Can you work these out from the model? Positions are in its coordinate system, mm. A direction names the side the tool comes from. Give positions to 0.01 mm unless a question says otherwise; leave off trailing zeros. Order: outer loops, then holes, each group sorted by start corner. A loop starts at its lowest first (then second) coordinate and runs counter-clockwise, first axis right, second up. Notation, with made-up numbers: (-16.75, 85) -> (32.25, 85) arc R7 cw to (32.25, 97) -> close; hole circle Ø9 at (-38, 74.25). An arc over 180 degrees is marked (long way). Answer as a JSON object with one key per item and string values.
```python
from build123d import *

# Parameters (mm, degrees)
SKETCH1_W           = 162.5727
SKETCH1_H           = 69.9897
BOSS_EXTRUDE1_DEPTH = 101.6635
SKETCH2_R           = 9.525
BOSS_EXTRUDE2_DEPTH = 69.9897
SKETCH3_W           = 34.9885
SKETCH3_H           = 22.29485
CUT_EXTRUDE1_DEPTH  = 1275.884686052
CUT_EXTRUDE2_DEPTH  = 27.432
CUT_EXTRUDE3_REACH  = 1269.087
CUT_EXTRUDE5_REACH  = 1269.087


with BuildPart() as part:
    # Sketch1 → Boss-Extrude1 (new body)
    with BuildSketch(Plane.XY):
        with Locations((634.389537826, 1225.388271401)):
            Rectangle(SKETCH1_W, SKETCH1_H)
    extrude(amount=BOSS_EXTRUDE1_DEPTH)

    # Sketch2 → Boss-Extrude2 (add, through all)
    with BuildSketch(Plane(origin=(0, 1260.383121401, 0), x_dir=(1, 0, 0), z_dir=(0, 1, 0))):
        Polygon((582.567187826, 0), (625.213787826, 34.9885), (643.565287826, 34.9885), (686.211887826, 0), align=None)
        with Locations(Location((634.389537826, 15.3035, 0), (0, 0, 270))):
            Circle(SKETCH2_R, mode=Mode.SUBTRACT)
    extrude(amount=-BOSS_EXTRUDE2_DEPTH)

    # Sketch3 → Cut-Extrude1 (cut, through all)
    with BuildSketch(Plane.ZY.offset(-553.103187826)):
        with Locations((-17.49425, 1201.540846401)):
            Rectangle(SKETCH3_W, SKETCH3_H)
        with Locations((-17.49425, 1249.235696401)):
            Rectangle(SKETCH3_W, SKETCH3_H)
    extrude(amount=-CUT_EXTRUDE1_DEPTH, mode=Mode.SUBTRACT)

    # Sketch5 → Cut-Extrude2 (cut, symmetric)
    with BuildSketch(Plane(origin=(0, 1225.388271401, 0), x_dir=(1, 0, 0), z_dir=(0, 1, 0))):
        Polygon((558.183187826, -101.6635), (561.485187826, -91.5035), (707.293887826, -91.5035), (710.595887826, -101.6635), align=None)
    extrude(amount=CUT_EXTRUDE2_DEPTH, both=True, mode=Mode.SUBTRACT)

    # Cut-Extrude3: up to this plane
    cut_extrude3_end = Plane(origin=(707.293887826, 1197.956271401, 91.5035), z_dir=(0.9510340687309474, 0, -0.3090860723375604))
    # Sketch6 → Cut-Extrude3 (cut, up to the surface)
    with BuildSketch(Plane.ZY.offset(-634.389537826), mode=Mode.PRIVATE) as cut_extrude3_sk1:
        Polygon((101.6635, 1255.303121401), (91.5035, 1252.820271401), (101.6635, 1252.820271401), align=None)
    cut_extrude3_tool1 = split(extrude(cut_extrude3_sk1.sketch, amount=-CUT_EXTRUDE3_REACH, mode=Mode.PRIVATE), bisect_by=cut_extrude3_end, keep=Keep.BOTH, mode=Mode.PRIVATE)
    add(cut_extrude3_tool1.solids().sort_by_distance((634.389538, 1253.647888, 98.276833))[0], mode=Mode.SUBTRACT)
    # Sketch6 → Cut-Extrude3 (cut, up to the surface)
    with BuildSketch(Plane.ZY.offset(-634.389537826), mode=Mode.PRIVATE) as cut_extrude3_sk2:
        Polygon((91.5035, 1197.956271401), (101.6635, 1195.473421401), (101.6635, 1197.956271401), align=None)
    cut_extrude3_tool2 = split(extrude(cut_extrude3_sk2.sketch, amount=-CUT_EXTRUDE3_REACH, mode=Mode.PRIVATE), bisect_by=cut_extrude3_end, keep=Keep.BOTH, mode=Mode.PRIVATE)
    add(cut_extrude3_tool2.solids().sort_by_distance((634.389538, 1197.128655, 98.276833))[0], mode=Mode.SUBTRACT)

    # Cut-Extrude5: up to this face of the body (flat: up to its plane)
    cut_extrude5_end = Plane(part.part.faces().sort_by_distance((559.834187826, 1225.388271401, 96.5835))[0])
    # Sketch8 → Cut-Extrude5 (cut, up to the picked face)
    with BuildSketch(Plane(origin=(634.389537826, 0, 0), x_dir=(0, 0, -1), z_dir=(1, 0, 0)), mode=Mode.PRIVATE) as cut_extrude5_sk1:
        Polygon((-101.6635, 1255.303121401), (-91.5035, 1252.820271401), (-91.5035, 1197.956271401), (-101.6635, 1195.473421401), align=None)
    cut_extrude5_tool1 = split(extrude(cut_extrude5_sk1.sketch, amount=-CUT_EXTRUDE5_REACH, mode=Mode.PRIVATE), bisect_by=cut_extrude5_end, keep=Keep.BOTH, mode=Mode.PRIVATE)
    add(cut_extrude5_tool1.solids().sort_by(Axis((634.389538, 1225.388271, 96.656813), (-1, 0, 0)))[0], mode=Mode.SUBTRACT)


solid = part.part
```
1. For faces 1 (the face through (645, 1212.688, -14)), 2 (the face through (645, 1238.088, -14)), 3 (the face through (640.83, 1225.57, -22.32)), 4 (the face through (708.92, 1224.97, 96.51)), which set-ups out of +Z, -Z, +X, -X, +Y, -Y let a thin tool reach every point of the face, with its end or its side?
Worked answers:
{"face 1": "-Z, +X, -X, -Y", "face 2": "-Z, +X, -X, +Y", "face 3": "+Y, -Y", "face 4": "+Z"}
2. If we mould it in two halves opening along Y, with no side actions, what happens to faces 5 (the face through (553.103, 1225, 50)), 6 (the face through (635.456, 1196.732, 96.512)), 7 (the face through (633, 1190.393, 50))? For each: +Y half, -Y half, draft (parallel to the pull), parting line (faces both ways), or undercut.
Worked answers:
{"face 5": "draft", "face 6": "undercut", "face 7": "-Y half"}
3. Please list where these lines run through material, in increasing order: L1, parallel to Z at x = 690.5, y = 1251.5; L2, parallel to Z at x = 673.5, y = 1194; L3, parallel to Y at x = 668.5, z = -11.
Worked answers:
{"L1": "0 to 91.5", "L2": "0 to 101.66", "L3": "1212.69 to 1238.09"}
4. If we section it at B-B on x = 698: Please give me the cut outline in (y, z).
Worked answers:
{"outline": "(1190.39, 0) -> (1260.38, 0) -> (1260.38, 101.66) -> (1255.3, 101.66) -> (1252.82, 91.5) -> (1197.96, 91.5) -> (1195.47, 101.66) -> (1190.39, 101.66) -> close"}
5. If we section it at A-A on y = 1201: Please give me the cut outline in (x, z), then the cut area to 3 significant figures.
Worked answers:
{"outline": "(553.1, 0) -> (715.68, 0) -> (715.68, 101.66) -> (710.6, 101.66) -> (707.29, 91.5) -> (561.49, 91.5) -> (558.18, 101.66) -> (553.1, 101.66) -> close", "area": "15,000 mm²"}
6. Will these pins go through, and if not, where does the flat tip stop? pin 1 Ø17.5 at (x, z) = (644, -25) entering from +Y; pin 2 Ø3 at (x, y) = (614.5, 1236.5) entering from -Z; pin 3 Ø10 at (x, y) = (609.5, 1251) entering from -Z.
Worked answers:
{"pin 1": "y = 1238.09", "pin 2": "z = -27.43", "pin 3": "z = 0"}
7. If we section it at D-D on x = 662: Please give me the cut outline in (y, z).
Worked answers:
{"outline": "(1190.39, 0) -> (1212.69, 0) -> (1212.69, -19.86) -> (1238.09, -19.86) -> (1238.09, 0) -> (1260.38, 0) -> (1260.38, 101.66) -> (1255.3, 101.66) -> (1252.82, 91.5) -> (1197.96, 91.5) -> (1195.47, 101.66) -> (1190.39, 101.66) -> close"}
